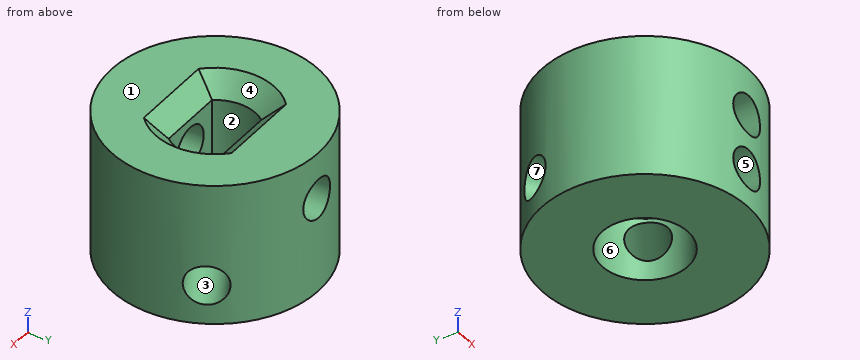
Autodesk Inventor part; units mm, degrees
ref_plane "Work Plane1" through (-20.8033, -6.3, -5.9) normal (0, 0, 1) x (1, 0, 0)
ref_plane "YZ Plane" through (0, 0, 0) normal (1, 0, 0) x (0, 1, 0)
ref_plane "XZ Plane" through (0, 0, 0) normal (0, 1, 0) x (-1, 0, 0)
sketch "Sketch1" plane through (0, 0, 0) normal (0, 0, 1) x (1, 0, 0)
  line L0 (0.8467, -0.7217) -> (0.8467, 0.7217) construction
  line L1 (0.8467, 0.7217) -> (2.0967, 1.4434) construction
  line L2 (2.0967, 1.4434) -> (3.3467, 0.7217) construction
  line L3 (3.3467, 0.7217) -> (3.3467, -0.7217) construction
  line L4 (3.3467, -0.7217) -> (2.0967, -1.4434) construction
  line L5 (2.0967, -1.4434) -> (0.8467, -0.7217) construction
  circle A0 centre (2.0967, 0) radius 2.45 construction
  line L6 (4.8467, -1.5877) -> (3.4717, -2.3816) construction
  line L7 (15.0967, 3) -> (15.0967, -3) construction
  line L8 (-10.9033, 3) -> (-10.9033, -3) construction
  line L9 (-0.6533, 0) -> (-0.6533, 1.5877) construction
  circle A1 centre (2.0967, 0) radius 5
  circle A2 centre (2.0967, 0) radius 1.7
  line L10 (-10.9033, -3) -> (15.0967, -3)
  line L11 (-10.9033, 3) -> (15.0967, 3)
  circle A3 centre (2.0967, 0) radius 2.7
  circle A4 centre (2.0967, 0) radius 6.5
  circle A5 centre (2.0967, 0) radius 2.75
  point P0 (0.4719, -0.5)
  point P1 (3.7215, -0.5)
  dimension "d10" = 5.4
  dimension "d13" = 13
ref_plane "Work Plane1" through (-20.8033, -6.3, -5.9) normal (0, 0, 1) x (1, 0, 0)
extrude "Extrusion1" add sketch "Sketch1" against normal blind 4 contours A1 L10 L11 | A1 L11 A4 L10 | L11 A1 | A1 L11 A4 | L10 A4 A1 | A1 L10 | A1 L10 A4 L11 | A5
sketch "Sketch2" plane through (2.0967, 0, 0) normal (0, 0, 1) x (1, 0, 0)
  line L0 (-2, 1.5) -> (2, 1.5) construction
  arc A0 (2.5, 0) -> (2, 1.5) centre (0, 0) ccw construction
  arc A1 (-2, 1.5) -> (-2.5, 0) centre (0, 0) ccw construction
  line L1 (2, -1.5) -> (-2, -1.5) construction
  arc A2 (-2.5, 0) -> (2.5, 0) centre (0, 0) ccw construction
  line L2 (2.0248, 1.55) -> (-2.0248, 1.55) construction
  arc A3 (-2.0248, 1.55) -> (-2.55, 0) centre (0, 0) ccw construction
  arc A4 (-2.55, 0) -> (2.55, 0) centre (0, 0) ccw construction
  arc A5 (2.55, 0) -> (2.0248, 1.55) centre (0, 0) ccw construction
  line L3 (-2.0248, 1.55) -> (2.0248, 1.55) construction
  line L4 (-2.0248, 1.55) -> (2.0248, 1.55)
  line L5 (-2.0248, -1.55) -> (2.0248, -1.55)
  arc A6 (-2.0248, 1.55) -> (-2.0248, -1.55) centre (0, 0) ccw
  arc A7 (2.0248, -1.55) -> (2.0248, 1.55) centre (0, 0) ccw
  circle A8 centre (0, 0) radius 6.5
  point P0 (-2.0967, 0)
  dimension "d11" = 3.1
  dimension "d12" = 2.55
extrude "Extrusion2" add sketch "Sketch2" along normal blind 5
chamfer "Chamfer1" distance 1.2 angle 45 4 edges at (2.0967, 1.55, 5) (-0.4533, 0, 5) (2.0967, -1.55, 5) (4.6467, 0, 5)
sketch "Sketch3" plane through (0, 0, 0) normal (0, 1, 0) x (-1, 0, 0)
  line L0 (-4.6467, 0) -> (-4.6467, 3.8)
  line L1 (0.4533, 0) -> (0.4533, 3.8)
  line L2 (-8.5967, -4) -> (4.4033, -4)
  circle A0 centre (-2.0967, -1.5) radius 1.25
  line L3 (-8.5967, -4) -> (4.4033, -4)
  point P0 (0, 0)
  point P1 (-8.5967, 0)
  point P2 (4.4033, 0)
  dimension "d14" = 2.5
  dimension "d15" = 2.5
extrude "Extrusion3" cut sketch "Sketch3" against normal blind 10
pattern_circular "Circular Pattern1" count 3 over 360 about axis through (2.0967, 0, 0) along (0, 0, -1) of "Extrusion3"
sketch "Sketch4" plane through (0.0718, -1.55, 0) normal (0, 1, 0) x (1, 0, 0)
  line L0 (0, -3.8) -> (4.0497, -3.8)
  line L1 (-4.4752, -5) -> (8.5248, -5)
  line L2 (8.5248, 4) -> (-4.4752, 4)
  line L3 (4.0497, -3.8) -> (0, -3.8)
  line L4 (4.0497, 0) -> (4.0497, -3.8)
  line L5 (0, 0) -> (4.0497, 0)
  line L6 (0, 0) -> (0, -3.8)
  circle A0 centre (2.0248, -2.0248) radius 2.0248
  point P0 (-0.0718, 0)
  point P1 (8.1739, 1.5)
  point P2 (-2.8742, 1.5)
  point P3 (0.7748, 1.5)
hole "Hole1" at (2.0967, -1.55, 2.0248) direction (0, -1, 0) diameter 2.5 end through all both
properties part number "30_Coupling_Screw_28BYJ_M3"
For this review, take the finished solid that the model builds, in its own axes (mm). Face numbers are marked on the shaded views. A direction names the side the tool comes from. Round coordinates to 2 decimals unless told otherwise and drop trailing zeros. Write each loop counter-clockwise with the first axis right and the second up, starting at its lowest first coordinate (ties: lowest second). Pieces come first, ordered by that corner, then holes. Notation, with made-up numbers: (5.5, 56.5) - (56.5, 56.5) arc R24 ccw to (56.5, 95.5) - close; hole circle Ø7 at (61, 43). An arc over 180 degrees is marked (long way). Write item = value, one per line. Start each with the question number.
1. Draft analysis for pull direction Z (two halves, no side actions). For the marked faces 1, 2 and 3, state which applies: released by +Z, released by -Z, zero draft, split by the parting line, or undercut.
2. Consider section B-B on z = -1.25. State the section outline as (x, y) points.
3. Consider section D-D on y = -3. State the section outline as (x, z) points.
4. Wall thickness on L1, parallel to Z at x = 1.5, y = -3.75; L2, parallel to X at y = -4.7, z = -1.5; L3, parallel to X at y = -2.5, z = -1: over which ranges is each line inside the solid? List them lowest first.
5. For the marked faces 4, 5, 6 and 7, list the 3-axis set-ups (+Z, -Z, +X, -X, +Y, -Y) from which the entire face can be reached by the end or side of a thin tool; tool diameter is ignored.
6. For pin 1 Ø3 at (x, z) = (2.1, 2.02) entering from -Y; pin 2 Ø4 at (x, z) = (-2, -3) entering from +Y; pin 3 Ø1.5 at (y, z) = (4, -1.5) entering from -X; pin 4 Ø3 at (y, z) = (3.5, 2) entering from -X, all flat-tipped, find the tip position at first contact; note any pin that passes through.
7. Consider section A-A on z = 3.5. State the section outline as (x, y) points.
8. Consider section C-C on z = 2. State the section outline as (x, y) points, plus the area to 3 significant figures.
Evaluation:
q1.face_1 = released by +Z
q1.face_2 = zero draft
q1.face_3 = undercut
q2.outline = (-4.04, 2.13) arc R6.5 ccw to (0.87, -6.38) - (0.87, -2.41) arc R2.7 cw to (-0.6, 0.14) - close; (-2.82, 4.25) - (0.63, 2.26) arc R2.7 cw to (3.57, 2.26) - (7.01, 4.25) arc R6.5 ccw to start; (3.32, -6.38) arc R6.5 ccw to (8.24, 2.13) - (4.79, 0.14) arc R2.7 cw to (3.32, -2.41) - close
q3.outline = (-3.67, -4) - (7.86, -4) - (7.86, 5) - (-3.67, 5) - close; hole circle Ø2.5 at (2.1, -1.5); hole circle Ø2.5 at (2.1, 2.02)
q4.L1 = -4 to -2.6, -0.4 to 0.93, 3.12 to 5
q4.L2 = -2.39 to 0.85, 3.35 to 6.59
q4.L3 = -3.9 to 0.95, 3.24 to 8.1
q5.face_4 = +Z
q5.face_5 = -Y
q5.face_6 = -Z
q5.face_7 = none
q6.pin_1 = -6.5
q6.pin_2 = 6.15
q6.pin_3 = -2.96
q6.pin_4 = -4.09
q7.outline = circle Ø13 at (2.1, 0); hole (0.07, -1.55) - (4.12, -1.55) arc R2.55 ccw to (4.12, 1.55) - (0.07, 1.55) arc R2.55 ccw to start
q8.outline = (0.07, -1.55) arc R2.55 cw to (0.07, 1.55) - (0.85, 1.55) - (0.85, 6.38) arc R6.5 ccw to (0.85, -6.38) - (0.85, -1.55) - close; (3.35, -6.38) arc R6.5 ccw to (3.35, 6.38) - (3.35, 1.55) - (4.12, 1.55) arc R2.55 cw to (4.12, -1.55) - (3.35, -1.55) - close
q8.area = 93.4 mm2
